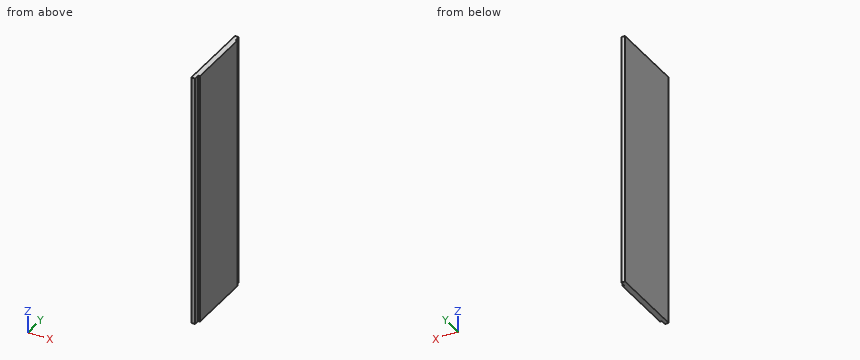
from build123d import *

# Parameters (mm, degrees)
F0_W     = 88.9
F0_H     = 298.45
F2_DEPTH = 4.233418
F1_W     = 76.2
F1_H     = 298.45
F3_DEPTH = 2.116455


with BuildPart() as f2:
    # F0 (on Right) → F2 (new body)
    with BuildSketch(Plane.YZ):
        with Locations((44.45, 149.225)):
            Rectangle(F0_W, F0_H)
    extrude(amount=-F2_DEPTH)

    # F1 (on Right) → F3 (join)
    with BuildSketch(Plane.YZ):
        with Locations((44.45, 149.225)):
            Rectangle(F1_W, F1_H)
    extrude(amount=F3_DEPTH)


solid = f2.part
Could you check a few things on this model? Use its own coordinates, in mm. Round coordinates to 2 decimals unless told otherwise and drop trailing zeros. Write each loop counter-clockwise with the first axis right and the second up, starting at its lowest first coordinate (ties: lowest second). Pieces come first, ordered by that corner, then holes. Notation, with made-up numbers: (-29, -39) -> (6, -39) arc R24 cw to (6, -4) -> close; hole circle Ø6 at (-27, -18.75). An arc over 180 degrees is marked (long way). Use a Markdown table: item, result.
1. Please list where these lines run through material, in increasing order: probe 1 along Y at (x, z) = (1.75, 35); probe 2 along X at (y, z) = (5, 69).
Answer key:
| item | result |
|---|---|
| probe 1 | y = 6.35 to 82.55 |
| probe 2 | x = -4.23 to 0 |
2. If we section it at A-A (z = 238.5): List the corners of the cut face in (x, y) for me.
Answer key:
| item | result |
|---|---|
| outline | (-4.23, 0) -> (0, 0) -> (0, 6.35) -> (2.12, 6.35) -> (2.12, 82.55) -> (0, 82.55) -> (0, 88.9) -> (-4.23, 88.9) -> close |
3. For pin 1 Ø0.6 at (x, z) = (1, 135) entering from -Y; pin 2 Ø5 at (y, z) = (86.5, 179.5) entering from +X, each with a flat end and sliding along its axis, tell me the tip position at first contact or that it passes through.
Answer key:
| item | result |
|---|---|
| pin 1 | stops at y = 6.35 |
| pin 2 | stops at x = 0 |
